The listing builds one solid part. Answer for the finished solid, in the listing's coordinates (mm). Face numbers are marked on the shaded views. A direction names the side the tool comes from. Give positions to 0.01 mm unless a question says otherwise; leave off trailing zeros. Loops run counter-clockwise (first coordinate to the right, second up) from the corner with the lowest first, then second, coordinate; pieces in that order, holes last. Notation, with made-up numbers: (53, 40) - (81, 40) arc R5 ccw to (81, 46) - close; hole circle Ø4 at (32.5, 45.5). An arc over 180 degrees is marked (long way). Answer as CSV lines item,"result". Start each with the question number.
1) For a pull along Z with two mould halves and no side action, classify the marked faces 1, 2, 3 and 4 as pulls with the +Z half, pulls with the -Z half, needs draft (parallel to the pull), parting line crosses it, or undercut.
2) Flat-ended cylindrical pins translate along their axes: pin 1 (5 mm diameter, centred on x = -45, y = 0, fed in from -Z); pin 2 (6 mm diameter, centred on x = -27, z = -3.5, fed in from -Y). Find the tip coordinate at first contact, or state that the pin passes through.
3) For the marked faces 5, 6 and 7, determine the directions among +Z, -Z, +X, -X, +Y, -Y from which every point of the face is accessible in a straight line to the end or side of a thin tool.
4) A cutting plane is placed at C-C (z = 0). Determine the outline of the cut face in (x, y), and give its area (3 significant figures).
5) A cutting plane is placed at B-B (x = -64). Determine the outline of the cut face in (y, z).
6) Find the intervals of material crossed by line 1 along Y through (x, z) = (-16, 0); line 2 along Z through (x, y) = (-15.75, 8.3); line 3 along Z through (x, y) = (-30.75, 8.3), in increasing order.
7) A cutting plane is placed at D-D (y = -1.25). Determine the outline of the cut face in (x, z), and give its area (3 significant figures).
8) A cutting plane is placed at A-A (x = -45). Determine the outline of the cut face in (y, z).
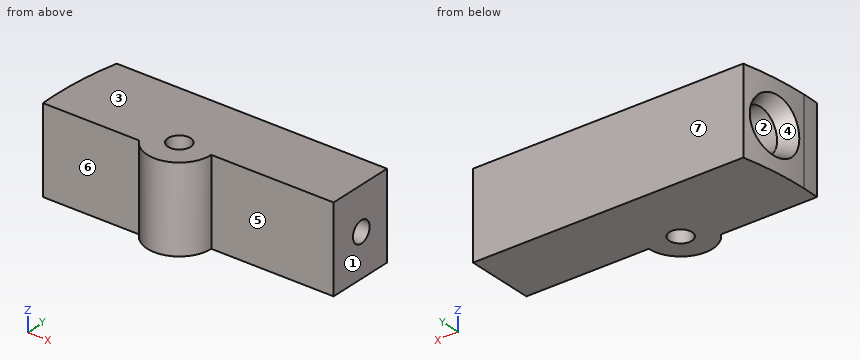
```python
from build123d import *

# Parameters (mm, degrees)
SKETCH2_R           = 2.65
BOSS_EXTRUDE1_DEPTH = 10
SKETCH4_R           = 75.7
SKETCH4_R_2         = 74
CUT_EXTRUDE5_DEPTH  = 80.915518032
SKETCH5_W           = 3
SKETCH5_H           = 16
CUT_EXTRUDE6_DEPTH  = 79.307087942


with BuildPart() as part:
    # Sketch2 → Boss-Extrude1 (new, symmetric)
    with BuildSketch(Plane.XY):
        with BuildLine():
            ThreePointArc((-73.989796594, 16), (-75.457580373, 6.053392794), (-75.594245813, -4))
            Line((-75.594245813, -4), (-51.34428877, -4))
            ThreePointArc((-51.34428877, -4), (-42.918193786, -7.205281597), (-37.5, 0))
            Line((-37.5, 0), (-5.763957799, 0))
            Line((-5.763957799, 0), (-5.763957799, 16))
            Line((-5.763957799, 16), (-73.989796594, 16))
        make_face()
        with Locations((-45, 0)):
            Circle(SKETCH2_R, mode=Mode.SUBTRACT)
    extrude(amount=BOSS_EXTRUDE1_DEPTH, both=True)

    # Sketch3 → Cut-Revolve1 (revolve, cut)
    with BuildSketch(Plane.XY, mode=Mode.PRIVATE) as cut_revolve1_sk:
        Polygon((-76.243604379, 8.3), (-75.243604379, 8.3), (-55.276091822, 8.3), (11.256395621, 8.3), (11.256395621, 10.8), (-23.743604379, 10.8), (-25.243604379, 12.3), (-48.243604379, 12.3), (-49.243604379, 13.3), (-70.243604379, 13.3), (-76.243604379, 13.3), align=None)
        Polygon((-76.243604379, 16.3), (-76.243604379, 13.3), (-70.243604379, 13.3), align=None)
    revolve(cut_revolve1_sk.sketch.rotate(Axis((-75.243604379, 8.3, 0), (1, 0, 0)), 90), axis=Axis((-75.243604379, 8.3, 0), (1, 0, 0)), mode=Mode.SUBTRACT)

    # Sketch4 → Cut-Extrude5 (cut, through all)
    with BuildSketch(Plane(origin=(0, 0, -10), x_dir=(-1, 0, 0), z_dir=(0, 0, -1))):
        Circle(SKETCH4_R)
        Circle(SKETCH4_R_2, mode=Mode.SUBTRACT)
    extrude(amount=-CUT_EXTRUDE5_DEPTH, mode=Mode.SUBTRACT)

    # Sketch5 → Cut-Extrude6 (cut, through all)
    with BuildSketch(Plane(origin=(0, 0, -10), x_dir=(-1, 0, 0), z_dir=(0, 0, -1))):
        with Locations((7.263957799, 8)):
            Rectangle(SKETCH5_W, SKETCH5_H)
    extrude(amount=-CUT_EXTRUDE6_DEPTH, mode=Mode.SUBTRACT)


solid = part.part
```
Ans:
1,face 1,"needs draft"
1,face 2,"undercut"
1,face 3,"pulls with the +Z half"
1,face 4,"undercut"
2,pin 1,"through"
2,pin 2,"y = 0"
3,face 5,"+Z, -Z, +X, -Y"
3,face 6,"+Z, -Z, -X, -Y"
3,face 7,"+Z, -Z, +X, -X, +Y"
4,outline,"(-73.99, 1.43) arc R74 ccw to (-73.89, -4) - (-51.34, -4) arc R7.5 ccw to (-37.5, 0) - (-8.76, 0) - (-8.76, 5.8) - (-23.74, 5.8) - (-25.24, 4.3) - (-48.24, 4.3) - (-49.24, 3.3) - (-70.24, 3.3) - close; (-72.57, 14.46) - (-70.24, 13.3) - (-49.24, 13.3) - (-48.24, 12.3) - (-25.24, 12.3) - (-23.74, 10.8) - (-8.76, 10.8) - (-8.76, 16) - (-72.25, 16) arc R74 ccw to start; hole circle Ø5.3 at (-45, 0)"
4,area,"663 mm2"
5,outline,"(-4, -10) - (16, -10) - (16, 10) - (-4, 10) - close; hole circle Ø10 at (8.3, 0)"
6,line 1,"0 to 5.8, 10.8 to 16"
6,line 2,"-10 to -2.5, 2.5 to 10"
6,line 3,"-10 to -4, 4 to 10"
7,outline,"(-73.99, -10) - (-47.34, -10) - (-47.34, 10) - (-73.99, 10) - close; (-42.66, -10) - (-37.6, -10) - (-37.6, 10) - (-42.66, 10) - close"
7,area,"634 mm2"
8,outline,"(-7.5, -10) - (-2.65, -10) - (-2.65, 10) - (-7.5, 10) - close; (2.65, -10) - (16, -10) - (16, 10) - (2.65, 10) - close; hole circle Ø8 at (8.3, 0)"
